Read the model definition and answer for the solid it produces. Units are mm, in the model's axes. A direction names the side the tool comes from. Coordinates: 2 decimals unless noted, no trailing zeros. Loops run counter-clockwise (first coordinate to the right, second up) from the corner with the lowest first, then second, coordinate; pieces in that order, holes last. Notation, with made-up numbers: M 62.25,-38 L 93.25,-38 A9 ccw 93.25,-23 Z; hole C -20,80 d5. An arc over 180 degrees is marked long. One line per item, written item: value. Start each with the question number.
1. Consider probe 1 along X at (y, z) = (-14, 12.25); probe 2 along Y at (x, z) = (9, 20.25); probe 3 along Y at (x, z) = (75.5, 20). Determine where each line is inside the solid, lowest interval first.
2. The part is cut by section B-B (x = -30). Write down the section's boundary in (y, z).
3. For faces 5 (the face through (-78, -10, 10)), 6 (the face through (-62.373, -31.759, 24.145)), 7 (the face through (-62.373, -31.759, 0.855)), determine the directions among +Z, -Z, +X, -X, +Y, -Y from which every point of the face is accessible in a straight line to the end or side of a thin tool.
4. The part is cut by section C-C (z = 20). Write down the section's boundary in (x, y), then the cut area to 3 significant figures.
5. Flat-ended cylindrical pins translate along their axes: pin 1 (9.5 mm diameter, centred on y = -40, z = 13.5, fed in from -X); pin 2 (1 mm diameter, centred on y = -28, z = 5.5, fed in from +X); pin 3 (5.5 mm diameter, centred on x = -83, z = 12, fed in from -Y). Find the tip coordinate at first contact, or state that the pin passes through.
6. The part is cut by section A-A (y = -15.5). Write down the section's boundary in (x, z), then the cut area to 3 significant figures.
7. Determine the mould class of faces 1 (the face through (68, 0, 12)), 2 (the face through (58.58, -10.9, 12.63)), 3 (the face through (47.725, -20, 12)), 4 (the face through (-92.42, -9.1, 12.63)) for opening direction X: +X half, -X half, draft (parallel to the pull), parting line (faces both ways), or undercut.
```python
from build123d import *

# Parameters (mm, degrees)
F0_W     = 30
F0_H     = 10
F0_W_2   = 10
F0_H_2   = 30
F1_DEPTH = 25
F3_DEPTH = 25
F5_DEPTH = 25
F6_R     = 3


with BuildPart() as f1:
    # F0 (on Top) → F1 (new body)
    with BuildSketch(Plane.XY):
        with Locations((-78.2751372457, -5)):
            Rectangle(F0_W, F0_H)
        with Locations((-58.2751372457, -25)):
            Rectangle(F0_W_2, F0_H_2)
        Polygon((47.7248627543, 0), (47.7248627543, -40), (57.7248627543, -40), (57.7248627543, -10), (87.7248627543, -10), (87.7248627543, 0), align=None)
        with Locations((-58.2751372457, -5)):
            Rectangle(F0_W_2, F0_H)
        Polygon((47.7248627543, -40), (-53.2751372457, -40), (-63.2751372457, -40), (-63.2751372457, -50), (57.7248627543, -50), (57.7248627543, -40), align=None)
    extrude(amount=F1_DEPTH)

    # F2 (on face) → F3 (cut)
    with BuildSketch(Plane.XZ.offset(10)):
        with BuildLine():
            Line((74.2613053135, 13.7803687993), (72.7248627543, 12.5))
            Line((72.7248627543, 12.5), (74.2613053135, 11.2196312007))
            ThreePointArc((74.2613053135, 11.2196312007), (74.6054059097, 11.8191494725), (74.7248627543, 12.5))
            ThreePointArc((74.7248627543, 12.5), (74.6054059097, 13.1808505275), (74.2613053135, 13.7803687993))
        make_face()
        with BuildLine():
            Line((71.1884201952, 13.7803687993), (72.7248627543, 12.5))
            Line((72.7248627543, 12.5), (74.2613053135, 13.7803687993))
            ThreePointArc((74.2613053135, 13.7803687993), (72.7248627543, 14.5), (71.1884201952, 13.7803687993))
        make_face()
        with BuildLine():
            ThreePointArc((71.1884201952, 13.7803687993), (70.7248627543, 12.5), (71.1884201952, 11.2196312007))
            Line((71.1884201952, 11.2196312007), (72.7248627543, 12.5))
            Line((72.7248627543, 12.5), (71.1884201952, 13.7803687993))
        make_face()
        with BuildLine():
            Line((72.7248627543, 12.5), (71.1884201952, 11.2196312007))
            ThreePointArc((71.1884201952, 11.2196312007), (72.7248627543, 10.5), (74.2613053135, 11.2196312007))
            Line((74.2613053135, 11.2196312007), (72.7248627543, 12.5))
        make_face()
    extrude(amount=-F3_DEPTH, mode=Mode.SUBTRACT)

    # F4 (on face) → F5 (cut)
    with BuildSketch(Plane.XZ.offset(10)):
        with BuildLine():
            ThreePointArc((-79.8115798048, 11.2196312007), (-78.2751372457, 10.5), (-76.7386946865, 11.2196312007))
            Line((-76.7386946865, 11.2196312007), (-78.2751372457, 12.5))
            Line((-78.2751372457, 12.5), (-79.8115798048, 11.2196312007))
        make_face()
        with BuildLine():
            Line((-78.2751372457, 12.5), (-76.7386946865, 11.2196312007))
            ThreePointArc((-76.7386946865, 11.2196312007), (-76.3945940903, 11.8191494725), (-76.2751372457, 12.5))
            ThreePointArc((-76.2751372457, 12.5), (-76.3945940903, 13.1808505275), (-76.7386946865, 13.7803687993))
            Line((-76.7386946865, 13.7803687993), (-78.2751372457, 12.5))
        make_face()
        with BuildLine():
            Line((-79.8115798048, 13.7803687993), (-78.2751372457, 12.5))
            Line((-78.2751372457, 12.5), (-76.7386946865, 13.7803687993))
            ThreePointArc((-76.7386946865, 13.7803687993), (-78.2751372457, 14.5), (-79.8115798048, 13.7803687993))
        make_face()
        with BuildLine():
            Line((-79.8115798048, 11.2196312007), (-78.2751372457, 12.5))
            Line((-78.2751372457, 12.5), (-79.8115798048, 13.7803687993))
            ThreePointArc((-79.8115798048, 13.7803687993), (-80.2751372457, 12.5), (-79.8115798048, 11.2196312007))
        make_face()
    extrude(amount=-F5_DEPTH, mode=Mode.SUBTRACT)

    # F6
    f6_edges = [f1.edges().sort_by_distance(p)[0] for p in [
        (-93.275137, -10, 12.5),
        (-78.275137, -10, 0),
        (-63.275137, -30, 0),
        (-63.275137, -30, 25),
        (-63.275137, -10, 12.5),
        (-78.275137, -10, 25),
        (-2.775137, -50, 0),
        (-2.775137, -50, 25),
        (-93.275137, -5, 0),
        (57.724863, -50, 12.5),
        (57.724863, -30, 0),
        (72.724863, -10, 0),
        (72.724863, -10, 25),
        (87.724863, -10, 12.5),
        (87.724863, -5, 0),
        (87.724863, -5, 25),
        (57.724863, -30, 25),
        (57.724863, -10, 12.5),
        (-93.275137, -5, 25),
    ]]
    fillet(f6_edges, radius=F6_R)


solid = f1.part
```
Answer block:
1. probe 1: x = -63.28 to -53.28, 47.72 to 57.72
1. probe 2: y = -50 to -40
1. probe 3: y = -10 to 0
2. outline: M -50,3 A3 ccw -47,0 L -40,0 L -40,25 L -47,25 A3 ccw -50,22 Z
3. face 5: +Z, -Z, -X, -Y
3. face 6: +Z, -X, -Y
3. face 7: -Z, -X, -Y
4. outline: M -93.28,-7 A3 ccw -90.28,-10 L -66.28,-10 A3 cw -63.28,-13 L -63.28,-50 L 54.72,-50 A3 ccw 57.72,-47 L 57.72,-13 A3 cw 60.72,-10 L 84.72,-10 A3 ccw 87.72,-7 L 87.72,0 L 47.72,0 L 47.72,-40 L -53.28,-40 L -53.28,0 L -93.28,0 Z
4. area: 2,610 mm2
5. pin 1: stops at x = -63.28
5. pin 2: stops at x = 57.72
5. pin 3: stops at y = -10
6. outline: M -63.28,3 A3 ccw -60.28,0 L -53.28,0 L -53.28,25 L -60.28,25 A3 ccw -63.28,22 Z; M 47.72,0 L 54.72,0 A3 ccw 57.72,3 L 57.72,22 A3 ccw 54.72,25 L 47.72,25 Z
6. area: 492 mm2
7. face 1: draft
7. face 2: +X half
7. face 3: undercut
7. face 4: -X half
